Geometry: final body of the model. Coordinates: model frame, mm. A direction names the side the tool comes from. Give positions to 0.01 mm unless a question says otherwise; leave off trailing zeros. Order: outer loops, then holes, each group sorted by start corner. A loop starts at its lowest first (then second) coordinate and runs counter-clockwise, first axis right, second up. Notation, with made-up numbers: (-6.5, 88.5) - (1.5, 88.5) arc R28 ccw to (1.5, 114.5) - close; hole circle Ø11 at (-11, 73.25). An arc over 180 degrees is marked (long way). Put each result on its own line as item: value. Start each with the question number.
1. Section A-A on y = -50. Return the cut outline in (x, z), plus the area to 3 significant figures.
2. Ray query, line 1 along X through (y, z) = (-59.5, 3.15); line 2 along Y through (x, z) = (3.5, 1.9); line 3 along Y through (x, z) = (6, 0.45). Return the intervals inside material, ascending. Write a range as from..to.
3. Section C-C on z = 0.9. Count the separate pieces of the cut face and the enclosed holes in it, plus the area to 3 significant figures.
4. Set-up query: faces 1 (the cylindrical face through (2.1, -64.14, 2.54)), 2 (the flat face through (-3, -38, 2)). Return all of +Z, -Z, +X, -X, +Y, -Y with unobstructed straight access to the full face (end or side cutting, diameter ignored); none if empty.
5. Section B-B on x = 5. Return the cut outline in (y, z), plus the area to 3 significant figures.
6. First-contact query: P1, Ø2, axis at x = 0, y = -30, coming from the +Z side; P2, Ø1.5, axis at y = -1, z = 1.5, coming from the -X side; P3, Ø2, axis at y = -31, z = 1, coming from the -X side; P4, Ø1.5, axis at y = -1.5, z = 3.5, coming from the +X side. Flat tips, straight axial feed; report the tip coordinate or a pass-through.
7. Mould query, pull axis Y, two halves, no side actions, for faces 3 (the cylindrical face through (-2.1, -64.14, 2.54)), 4 (the cylindrical face through (-0.27, -21.22, 2.54)), 5 (the flat face through (3, -39, 2)). Classes: pulls with the +Y half, pulls with the -Y half, needs draft (parallel to the pull), parting line crosses it, or undercut.
from build123d import *

# Parameters (mm, degrees)
ESQUISSE1_R             = 15
ESQUISSE1_R_2           = 1.45
ESQUISSE1_R_3           = 1.498803823
ESQUISSE1_R_4           = 7.5
BOSS_EXTRU_1_DEPTH      = 5
CONG_1_R                = 3
CONG_2_R                = 3
ENL_V_MAT_EXTRU_1_REACH = 68.895
ESQUISSE2_R             = 1.25


with BuildPart() as part:
    # Esquisse1 → Boss.-Extru.1 (new body)
    # profile 1 of 3: a face of its own
    with BuildSketch(Plane.XY):
        with BuildLine():
            ThreePointArc((3, -14.696938457), (1.50763443, -14.924042295), (0, -15))
            Line((0, -15), (0, -65))
            Line((0, -65), (3, -65))
            Line((3, -65), (3, -14.696938457))
        make_face()
    # profile 2 of 3: a face of its own
    with BuildSketch(Plane.XY):
        with BuildLine():
            Line((0, -65), (0, -15))
            ThreePointArc((0, -15), (-1.50763443, -14.924042295), (-3, -14.696938457))
            Line((-3, -14.696938457), (-3, -65))
            Line((-3, -65), (0, -65))
        make_face()
    # profile 3 of 3: a face of its own
    with BuildSketch(Plane.XY):
        Circle(ESQUISSE1_R)
        with Locations((10.002593414, -5.775)):
            Circle(ESQUISSE1_R_2, mode=Mode.SUBTRACT)
        with Locations((0, 11.55)):
            Circle(ESQUISSE1_R_3, mode=Mode.SUBTRACT)
        with Locations((-10.002593414, -5.775)):
            Circle(ESQUISSE1_R_2, mode=Mode.SUBTRACT)
        Circle(ESQUISSE1_R_4, mode=Mode.SUBTRACT)
    extrude(amount=BOSS_EXTRU_1_DEPTH)

    # Congé1
    cong_1_edges = [part.edges().sort_by_distance(p)[0] for p in [
        (3, -65, 2.5),
    ]]
    fillet(cong_1_edges, radius=CONG_1_R)

    # Congé2
    cong_2_edges = [part.edges().sort_by_distance(p)[0] for p in [
        (-3, -65, 2.5),
    ]]
    fillet(cong_2_edges, radius=CONG_2_R - 0.0001)  # a hair under: the kernel refuses the full size

    # Esquisse2 → Enlèv. mat.-Extru.1 (cut, up to next)
    with BuildSketch(Plane.XY.offset(5), mode=Mode.PRIVATE) as enl_v_mat_extru_1_sk1:
        with Locations((0, -20)):
            Circle(ESQUISSE2_R)
    enl_v_mat_extru_1_tool1 = extrude(enl_v_mat_extru_1_sk1.sketch, amount=-ENL_V_MAT_EXTRU_1_REACH, mode=Mode.PRIVATE) & part.part
    # Esquisse2 → Enlèv. mat.-Extru.1 (cut, up to next)
    with BuildSketch(Plane.XY.offset(5), mode=Mode.PRIVATE) as enl_v_mat_extru_1_sk2:
        with Locations((0, -30)):
            Circle(ESQUISSE2_R)
    enl_v_mat_extru_1_tool2 = extrude(enl_v_mat_extru_1_sk2.sketch, amount=-ENL_V_MAT_EXTRU_1_REACH, mode=Mode.PRIVATE) & part.part
    # Esquisse2 → Enlèv. mat.-Extru.1 (cut, up to next)
    with BuildSketch(Plane.XY.offset(5), mode=Mode.PRIVATE) as enl_v_mat_extru_1_sk3:
        with Locations((0, -50)):
            Circle(ESQUISSE2_R)
    enl_v_mat_extru_1_tool3 = extrude(enl_v_mat_extru_1_sk3.sketch, amount=-ENL_V_MAT_EXTRU_1_REACH, mode=Mode.PRIVATE) & part.part
    # Esquisse2 → Enlèv. mat.-Extru.1 (cut, up to next)
    with BuildSketch(Plane.XY.offset(5), mode=Mode.PRIVATE) as enl_v_mat_extru_1_sk4:
        with Locations((0, -62)):
            Circle(ESQUISSE2_R)
    enl_v_mat_extru_1_tool4 = extrude(enl_v_mat_extru_1_sk4.sketch, amount=-ENL_V_MAT_EXTRU_1_REACH, mode=Mode.PRIVATE) & part.part
    add(enl_v_mat_extru_1_tool1.solids().sort_by_distance((0, -20, 5))[0], mode=Mode.SUBTRACT)
    add(enl_v_mat_extru_1_tool2.solids().sort_by_distance((0, -30, 5))[0], mode=Mode.SUBTRACT)
    add(enl_v_mat_extru_1_tool3.solids().sort_by_distance((0, -50, 5))[0], mode=Mode.SUBTRACT)
    add(enl_v_mat_extru_1_tool4.solids().sort_by_distance((0, -62, 5))[0], mode=Mode.SUBTRACT)


solid = part.part
Resolved:
1. outline: (-3, 0) - (-1.25, 0) - (-1.25, 5) - (-3, 5) - close; (1.25, 0) - (3, 0) - (3, 5) - (1.25, 5) - close
1. area: 17.5 mm^2
2. line 1: -3..3
2. line 2: -14.59..-6.63, 6.63..14.59
2. line 3: -13.75..-4.5, 4.5..13.75
3. separate pieces: 1
3. enclosed holes: 8
3. area: 787 mm^2
4. face 1: +Z, -Z, +X, -Y
4. face 2: +Z, -Z, -X, -Y
5. outline: (-14.14, 0) - (-5.59, 0) - (-5.59, 5) - (-14.14, 5) - close; (5.59, 0) - (14.14, 0) - (14.14, 5) - (5.59, 5) - close
5. area: 85.5 mm^2
6. P1: through
6. P2: x = -15
6. P3: x = -3
6. P4: x = 14.98
7. face 3: pulls with the -Y half
7. face 4: undercut
7. face 5: needs draft
